Work out the finished part from the listing and answer in its coordinate system (mm). Coordinates: 2 decimals unless noted, no trailing zeros. Order: outer loops, then holes, each group sorted by start corner. A loop starts at its lowest first (then second) coordinate and runs counter-clockwise, first axis right, second up. Notation, with made-up numbers: (68, -23) -> (99, -23) arc R11 ccw to (99, -12) -> close; hole circle Ø7 at (16, -35). An arc over 180 degrees is marked (long way). Write item = value, one per line. Start each with the question number.
Q1. The part is cut by section C-C, the plane x = 11.5. Determine the outline of the cut face in (y, z) (1 decimal).
Q2. The part is cut by section B-B, the plane y = 103.5. Determine the outline of the cut face in (x, z), plus the area to 3 significant figures.
Q3. The part is cut by section D-D, the plane y = -113.5. Determine the outline of the cut face in (x, z), plus the area to 3 significant figures.
Q4. For a pull along Y with two mould halves and no side action, classify faces 1 (the flat face through (30, -31, 2)), 2 (the cylindrical face through (15, 32, -24)), 3 (the cylindrical face through (14.79, 148.724, 19.527)) as +Y half, -Y half, draft (parallel to the pull), parting line (faces both ways), or undercut.
Q5. Straight lines are drawn through the part: L1, parallel to Y at x = 20, z = 0; L2, parallel to Z at x = 20, y = 62; L3, parallel to Y at x = 15.5, z = 36. For each, find the intervals that lie inside material, in ascending order. Write a range as from..to.
Q6. Flat-ended cylindrical pins translate along their axes: pin 1 (9 mm diameter, centred on x = 17, y = 67, fed in from +Z); pin 2 (6 mm diameter, centred on x = 8, z = 110, fed in from -Y); pin 3 (2 mm diameter, centred on x = 6.5, y = 34.5, fed in from -Z). Find the tip coordinate at first contact, or state that the pin passes through.
Q7. The part is cut by section A-A, the plane z = 0. Determine the outline of the cut face in (x, y), plus the area to 3 significant figures.
```python
from build123d import *

# Parameters (mm, degrees)
SKETCH1_R           = 150
SKETCH1_R_2         = 20
BOSS_EXTRUDE1_DEPTH = 30


with BuildPart() as part:
    # Sketch1 → Boss-Extrude1 (new body)
    with BuildSketch(Plane(origin=(0, 0, 0), x_dir=(0, 0, -1), z_dir=(1, 0, 0))):
        Circle(SKETCH1_R)
        Circle(SKETCH1_R_2, mode=Mode.SUBTRACT)
        with BuildLine():
            Line((110.639648089, 46.463623091), (33.744090545, 21.478741892))
            ThreePointArc((33.744090545, 21.478741892), (23.511410092, 32.360679775), (10, 38.729833462))
            Line((10, 38.729833462), (10, 119.582607431))
            ThreePointArc((10, 119.582607431), (70.534230275, 97.082039325), (110.639648089, 46.463623091))
        make_face(mode=Mode.SUBTRACT)
        with BuildLine():
            Line((-10, 119.582607431), (-10, 38.729833462))
            ThreePointArc((-10, 38.729833462), (-23.511410092, 32.360679775), (-33.744090545, 21.478741892))
            Line((-33.744090545, 21.478741892), (-110.639648089, 46.463623091))
            ThreePointArc((-110.639648089, 46.463623091), (-70.534230275, 97.082039325), (-10, 119.582607431))
        make_face(mode=Mode.SUBTRACT)
        with BuildLine():
            Line((116.819987977, 27.442492765), (39.924430433, 2.457611566))
            ThreePointArc((39.924430433, 2.457611566), (38.042260652, -12.360679775), (30.854994877, -25.455240937))
            Line((30.854994877, -25.455240937), (78.379063022, -90.86650912))
            ThreePointArc((78.379063022, -90.86650912), (114.126781955, -37.082039325), (116.819987977, 27.442492765))
        make_face(mode=Mode.SUBTRACT)
        with BuildLine():
            Line((62.198723135, -102.622214166), (14.674654989, -37.210945983))
            ThreePointArc((14.674654989, -37.210945983), (0, -40), (-14.674654989, -37.210945983))
            Line((-14.674654989, -37.210945983), (-62.198723135, -102.622214166))
            ThreePointArc((-62.198723135, -102.622214166), (0, -120), (62.198723135, -102.622214166))
        make_face(mode=Mode.SUBTRACT)
        with BuildLine():
            Line((-78.379063022, -90.86650912), (-30.854994877, -25.455240937))
            ThreePointArc((-30.854994877, -25.455240937), (-38.042260652, -12.360679775), (-39.924430433, 2.457611566))
            Line((-39.924430433, 2.457611566), (-116.819987977, 27.442492765))
            ThreePointArc((-116.819987977, 27.442492765), (-114.126781955, -37.082039325), (-78.379063022, -90.86650912))
        make_face(mode=Mode.SUBTRACT)
    extrude(amount=BOSS_EXTRUDE1_DEPTH)


solid = part.part
```
Model answer:
q1.outline = circle Ø300 at (0, 0); hole (-102.6, -62.2) -> (-37.2, -14.7) arc R40 cw to (-37.2, 14.7) -> (-102.6, 62.2) arc R120 ccw to start; hole (-90.9, -78.4) arc R120 ccw to (27.4, -116.8) -> (2.5, -39.9) arc R40 cw to (-25.5, -30.9) -> close; hole (-90.9, 78.4) -> (-25.5, 30.9) arc R40 cw to (2.5, 39.9) -> (27.4, 116.8) arc R120 ccw to start; hole circle Ø40 at (0, 0); hole (21.5, -33.7) -> (46.5, -110.6) arc R120 ccw to (119.6, -10) -> (38.7, -10) arc R40 cw to start; hole (21.5, 33.7) arc R40 cw to (38.7, 10) -> (119.6, 10) arc R120 ccw to (46.5, 110.6) -> close
q2.outline = (0, -108.57) -> (30, -108.57) -> (30, -60.73) -> (0, -60.73) -> close; (0, -10) -> (30, -10) -> (30, 10) -> (0, 10) -> close; (0, 60.73) -> (30, 60.73) -> (30, 108.57) -> (0, 108.57) -> close
q2.area = 3,470 mm2
q3.outline = (0, -98.07) -> (30, -98.07) -> (30, -38.96) -> (0, -38.96) -> close; (0, 38.96) -> (30, 38.96) -> (30, 98.07) -> (0, 98.07) -> close
q3.area = 3,550 mm2
q4.face_1 = draft
q4.face_2 = undercut
q4.face_3 = parting line
q5.L1 = -150..-120, -40..-20, 20..150
q5.L2 = -136.59..-102.74, -10..10, 102.74..136.59
q5.L3 = -145.62..-114.47, -66.56..-32.54, -17.44..22.21, 114.47..145.62
q6.pin_1 = 136.36
q6.pin_2 = -105.12
q6.pin_3 = -146.21
q7.outline = (0, -150) -> (30, -150) -> (30, -120) -> (0, -120) -> close; (0, -40) -> (30, -40) -> (30, -20) -> (0, -20) -> close; (0, 20) -> (30, 20) -> (30, 150) -> (0, 150) -> close
q7.area = 5,400 mm2
